For this review, use the dimensioned drawing (mm, ordinates from the lowest corner) and the shaded views. A direction names the side the tool comes from. Round coordinates to 2 decimals unless told otherwise and drop trailing zeros. Order: outer loops, then holes, each group sorted by start corner. A loop starts at its lowest first (then second) coordinate and runs counter-clockwise, first axis right, second up. Notation, with made-up numbers: M 27.5,51.25 L 48.5,51.25 A23 ccw 48.5,88.25 Z; hole C 69,-33 d9. An arc over 180 degrees is marked long. Use a Markdown table: item, result. Add a question column.
1. For the marked faces 1 and 2, list the 3-axis set-ups (+Z, -Z, +X, -X, +Y, -Y) from which the entire face can be reached by the end or side of a thin tool; tool diameter is ignored.
2. To check wall thickness, follow probe 1 along Z at (x, y) = (25, 74); probe 2 along X at (y, z) = (46.5, 188.5); probe 3 along Y at (x, z) = (45, 234.5). State the ranges of each line that lie inside material, in increasing order.
3. Consider section A-A on x = 44.45. State the section outline as (y, z) points.
4. Consider section B-B on z = 186.5. State the section outline as (x, y) points.
5. Insertion check: P1, Ø1, axis at x = 55.5, z = 63, coming from the -Y side; P2, Ø12, axis at y = 27.5, z = 374.5, coming from the -X side; P3, Ø3, axis at y = 21, z = 384.5, coming from the +X side. Each pin has a flat end and moves straight along its axis. Give the tip position at first contact, or say it passes through.
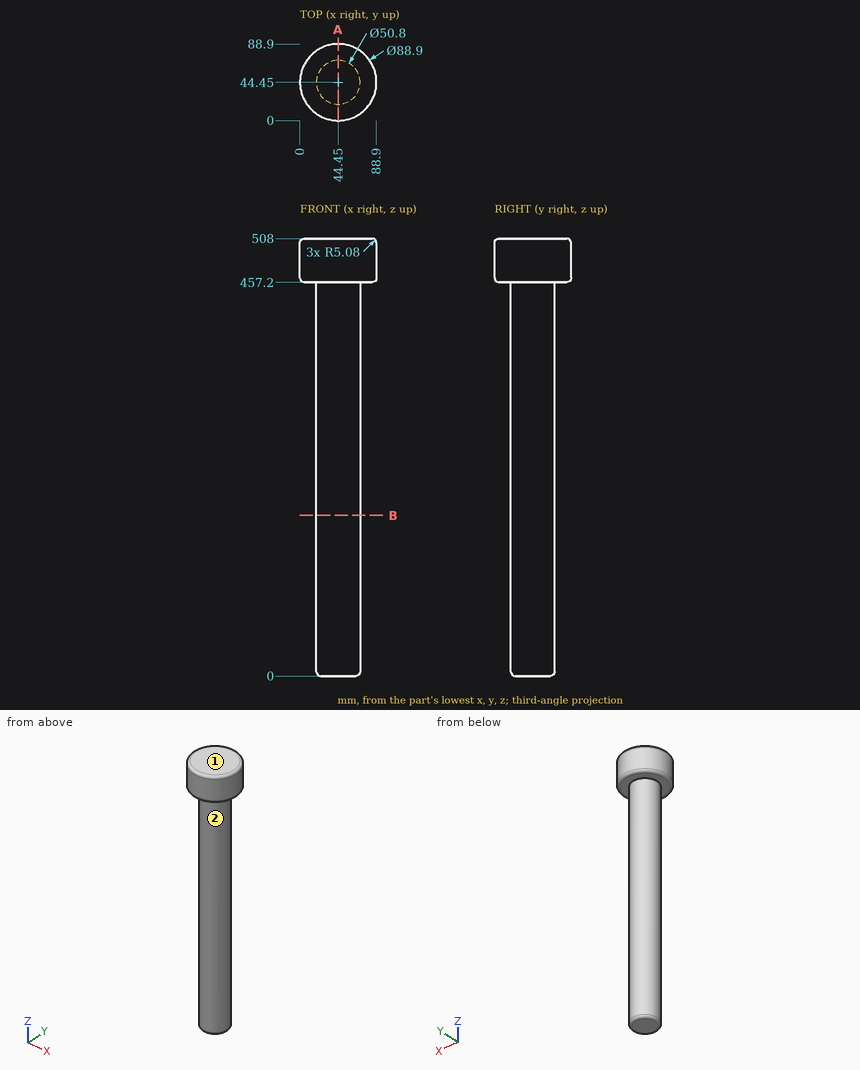
Answer block:
| question | item | result |
|---|---|---|
| 1 | face 1 | +Z, +X, -X, +Y, -Y |
| 1 | face 2 | -Z |
| 2 | probe 1 | 457.2 to 508 |
| 2 | probe 2 | 19.13 to 69.77 |
| 2 | probe 3 | 19.06 to 69.84 |
| 3 | outline | M 0,462.28 A5.08 ccw 5.08,457.2 L 19.05,457.2 L 19.05,5.08 A5.08 ccw 24.13,0 L 64.77,0 A5.08 ccw 69.85,5.08 L 69.85,457.2 L 83.82,457.2 A5.08 ccw 88.9,462.28 L 88.9,502.92 A5.08 ccw 83.82,508 L 5.08,508 A5.08 ccw 0,502.92 Z |
| 4 | outline | C 44.45,44.45 d50.8 |
| 5 | P1 | y = 21.34 |
| 5 | P2 | x = 21.53 |
| 5 | P3 | x = 57.23 |
